```python
from build123d import *

# Parameters (mm, degrees)
F0_R     = 3.175
F1_DEPTH = 25.4


with BuildPart() as f1:
    # F0 (on Front) → F1 (new body)
    with BuildSketch(Plane.XZ):
        Polygon((1476.254213, -1410.792774), (1730.254213, -1410.792774), (570.064314, 100.507226), (511.054213, 100.507226), (511.054213, -153.492774), align=None)
        with Locations((1035.730981, -737.692774)):
            Circle(F0_R, mode=Mode.SUBTRACT)
        with Locations((1086.530981, -737.692774)):
            Circle(F0_R, mode=Mode.SUBTRACT)
        with Locations((1386.712799, -1194.892774)):
            Circle(F0_R, mode=Mode.SUBTRACT)
        with Locations((1437.512799, -1194.892774)):
            Circle(F0_R, mode=Mode.SUBTRACT)
        with Locations((1488.312799, -1194.892774)):
            Circle(F0_R, mode=Mode.SUBTRACT)
        with Locations((1211.22189, -966.292774)):
            Circle(F0_R, mode=Mode.SUBTRACT)
        with Locations((1262.02189, -966.292774)):
            Circle(F0_R, mode=Mode.SUBTRACT)
        with Locations((1312.82189, -966.292774)):
            Circle(F0_R, mode=Mode.SUBTRACT)
        with Locations((1137.330981, -737.692774)):
            Circle(F0_R, mode=Mode.SUBTRACT)
        with Locations((684.749162, -280.492774)):
            Circle(F0_R, mode=Mode.SUBTRACT)
        with Locations((735.549162, -280.492774)):
            Circle(F0_R, mode=Mode.SUBTRACT)
        with Locations((786.349162, -280.492774)):
            Circle(F0_R, mode=Mode.SUBTRACT)
        with Locations((860.240072, -509.092774)):
            Circle(F0_R, mode=Mode.SUBTRACT)
        with Locations((911.040072, -509.092774)):
            Circle(F0_R, mode=Mode.SUBTRACT)
        with Locations((961.840072, -509.092774)):
            Circle(F0_R, mode=Mode.SUBTRACT)
        with Locations((547.358253, -51.892774)):
            Circle(F0_R, mode=Mode.SUBTRACT)
        with Locations((610.858253, -51.892774)):
            Circle(F0_R, mode=Mode.SUBTRACT)
    extrude(amount=F1_DEPTH)


solid = f1.part
```
Geometry check sheet. Reference: the model listing, model coordinates, mm. Round coordinates to 2 decimals unless told otherwise and drop trailing zeros. Loops run counter-clockwise (first coordinate to the right, second up) from the corner with the lowest first, then second, coordinate; pieces in that order, holes last. Notation, with made-up numbers: (-17, -20) - (-8, -20) arc R36 ccw to (-8, 14) - close; hole circle Ø10 at (6.5, 30.25). An arc over 180 degrees is marked (long way). Use a Markdown table: item, result.
Q1. Cross-section at C-C on x = 1168. Record the cut outline in (y, z).
Solutions:
| item | result |
|---|---|
| outline | (-25.4, -1009.25) - (0, -1009.25) - (0, -678.38) - (-25.4, -678.38) - close |
Q2. Material ranges on line 1 (X direction, y = -17.75, z = -966); line 2 (X direction, y = -8, z = -848); line 3 (X direction, y = -4.25, z = -571.5), recorded low to high.
Solutions:
| item | result |
|---|---|
| line 1 | x = 1134.8 to 1208.06, 1214.38 to 1258.86, 1265.18 to 1309.66, 1315.98 to 1388.8 |
| line 2 | x = 1044.21 to 1298.21 |
| line 3 | x = 831.95 to 1085.95 |
Q3. Cross-section at B-B on z = -127.5. Record the cut outline in (x, y), plus the area to 3 significant figures.
Solutions:
| item | result |
|---|---|
| outline | (511.05, -25.4) - (745.1, -25.4) - (745.1, 0) - (511.05, 0) - close |
| area | 5,940 mm2 |
Q4. Cross-section at A-A on y = -10.5. State how many separate pieces and enclosed holes the cut face has, plus the area to 3 significant figures.
Solutions:
| item | result |
|---|---|
| separate pieces | 1 |
| enclosed holes | 17 |
| area | 359,000 mm2 |
Q5. Go/stop test with flat-tipped pins: P1, Ø4, axis at y = -22, z = -902, coming from the -X side; P2, Ø10, axis at y = -5, z = -1108.5, coming from the -X side; P3, Ø10, axis at y = -12, z = -1164.5, coming from the +X side; P4, Ø7.5, axis at x = 1386.71, z = -1194.89, coming from the +Y side. Record where each tip stops, or that it passes through.
Solutions:
| item | result |
|---|---|
| P1 | stops at x = 1084.13 |
| P2 | stops at x = 1240.35 |
| P3 | stops at x = 1545.02 |
| P4 | stops at y = 0 |
